Input: part model. Units: mm. Frame: model coordinates. A direction names the side the tool comes from. Coordinates: 2 decimals unless noted, no trailing zeros. Loops run counter-clockwise (first coordinate to the right, second up) from the corner with the lowest first, then second, coordinate; pieces in that order, holes last.
Autodesk Inventor part; units mm, degrees
ref_plane "YZ Plane" through (0, 0, 0) normal (1, 0, 0) x (0, 1, 0)
ref_plane "XZ Plane" through (0, 0, 0) normal (0, 1, 0) x (-1, 0, 0)
ref_plane "XY Plane" through (0, 0, 0) normal (0, 0, 1) x (1, 0, 0)
sketch "Sketch1" plane through (0, 0, 0) normal (0, 1, 0) x (-1, 0, 0)
  line L0 (-425.45, 958.85) -> (425.45, 958.85)
  line L1 (425.45, 958.85) -> (425.45, -958.85)
  line L2 (425.45, -958.85) -> (-425.45, -958.85)
  line L3 (-425.45, -958.85) -> (-425.45, 958.85)
  line L4 (-425.45, 958.85) -> (425.45, -958.85) construction
  line L5 (425.45, 958.85) -> (-425.45, -958.85) construction
  point P0 (0, 0)
  dimension "d0" = 850.9
  dimension "d1" = 1917.7
extrude "Extrusion1" add sketch "Sketch1" along normal blind 3.175
sketch "Sketch2" plane through (0, 0, 0) normal (0, -1, 0) x (1, 0, 0)
  line L0 (425.45, -958.85) -> (-425.45, -958.85)
  line L1 (425.45, 958.85) -> (425.45, -958.85)
  line L2 (-425.45, 958.85) -> (425.45, 958.85)
  line L3 (-425.45, -958.85) -> (-425.45, 958.85)
  line L4 (-425.45, 958.85) -> (425.45, 958.85)
  line L5 (425.45, -958.85) -> (-425.45, -958.85)
  line L6 (425.45, 958.85) -> (422.275, 958.85)
  line L7 (422.275, 958.85) -> (422.275, -958.85)
  line L8 (422.275, -958.85) -> (425.45, -958.85)
  line L9 (425.45, -958.85) -> (425.45, 958.85)
  line L10 (-425.45, -958.85) -> (-425.45, 958.85)
  line L11 (-425.45, 958.85) -> (-422.275, 958.85)
  line L12 (-422.275, 958.85) -> (-422.275, -958.85)
  line L13 (-422.275, -958.85) -> (-425.45, -958.85)
  line L14 (-425.45, -958.85) -> (-425.45, 958.85)
  point P0 (0, 0)
  point P1 (-422.275, 958.85)
  point P2 (422.275, -958.85)
  dimension "d4" = 3.175
  dimension "d5" = 3.175
extrude "Extrusion2" add sketch "Sketch2" along normal blind 50.8 contours L0 L7 L2 L1 | L0 L3 L2 L12
fillet "Fillet1" radius 3.175 2 edges at (-422.275, 0, 0) (425.45, 3.175, 0)
properties part number "IronFrame" material "Iron, Cast"
Item 1: Reachability of faces 4 (the face through (425.45, -26, -13)), 5 (the face through (422.275, -25, 13)) from +Z, -Z, +X, -X, +Y, -Y: full face, straight path, thin tool, end or side. Return the list, or none.
Result:
face 4: +Z, -Z, +X, +Y, -Y
face 5: +Z, -Z, -Y
Item 2: Section query C-C (x = 203). Output: boundary loops of the cut face in (y, z) (3 decimals), then the cut area to 3 significant figures.
Result:
outline: (0, -958.85) - (3.175, -958.85) - (3.175, 958.85) - (0, 958.85) - close
area: 6,090 mm2
Item 3: Line query: L1, parallel to X at y = -11, z = 292 (3 decimals); L2, parallel to X at y = -2.5, z = 56.5 (3 decimals); L3, parallel to Y at x = 198.5, z = -15.5 (3 decimals). Output: solid intervals per line, ascending.
Result:
L1: x = -425.45 to -422.275, 422.275 to 425.45
L2: x = -425.45 to -422.202, 422.275 to 425.45
L3: y = 0 to 3.175
Item 4: Contact query for a flat-ended pin moving along its axis: P1, Ø5, axis at x = -119, z = -104.5, coming from the -Y side. Output: stop coordinate, or through.
Result:
P1: stops at y = 0
Item 5: Section query B-B (z = -481.5). Output: boundary loops of the cut face in (x, y) (3 decimals).
Result:
outline: (-425.45, -50.8) - (-422.275, -50.8) - (-422.275, -3.175) arc R3.175 cw to (-419.1, 0) - (422.275, 0) - (422.275, -50.8) - (425.45, -50.8) - (425.45, 0) arc R3.175 ccw to (422.275, 3.175) - (-425.45, 3.175) - close
Item 6: Mould query, pull axis X, two halves, no side actions, for faces 1 (the face through (2, 2, 958.85)), 2 (the face through (-425.45, -24, 13)), 3 (the face through (-422.275, -27, 13)). Classes: +X half, -X half, draft (parallel to the pull), parting line (faces both ways), or undercut.
Result:
face 1: draft
face 2: -X half
face 3: undercut
Item 7: Section query A-A (y = -34.5). Output: boundary loops of the cut face in (x, z) (3 decimals), then the cut area to 3 significant figures.
Result:
outline: (-425.45, -958.85) - (-422.275, -958.85) - (-422.275, 958.85) - (-425.45, 958.85) - close; (422.275, -958.85) - (425.45, -958.85) - (425.45, 958.85) - (422.275, 958.85) - close
area: 12,200 mm2
